Geometry: see drawing. Coordinates: mm, zero at the bounding-box minimum. A direction names the side the tool comes from. Round coordinates to 2 decimals unless told otherwise and drop trailing zeros. Loops run counter-clockwise (first coordinate to the right, second up) from the corner with the lowest first, then second, coordinate; pieces in that order, holes last.
(1) First-contact query: pin 1 Ø1.5 at (y, z) = (4, 6) entering from +X; pin 2 Ø6 at (x, z) = (7.5, 14.5) entering from -Y; pin 3 Ø1 at (x, z) = (1.5, 9.5) entering from +Y; pin 4 Ø1 at (x, z) = (7.5, 10.5) entering from -Y. Flat tips, straight axial feed; report the tip coordinate or a pass-through.
(2) Mould query, pull axis Y, two halves, no side actions, for the marked faces 3, 4, 5 and 6. Classes: pulls with the +Y half, pulls with the -Y half, needs draft (parallel to the pull), parting line crosses it, or undercut.
(3) Set-up query: the marked faces 1 and 2. Return all of +Z, -Z, +X, -X, +Y, -Y with unobstructed straight access to the full face (end or side cutting, diameter ignored); none if empty.
(4) Section C-C, the plane z = 6.25. Return the cut outline in (x, y), plus the area to 3 significant figures.
(5) Material intervals for probe 1 along Y at (x, z) = (5, 4.75); probe 2 along Y at (x, z) = (5, 9.75); probe 3 along Z at (x, y) = (3.5, 9), sorted ascending.
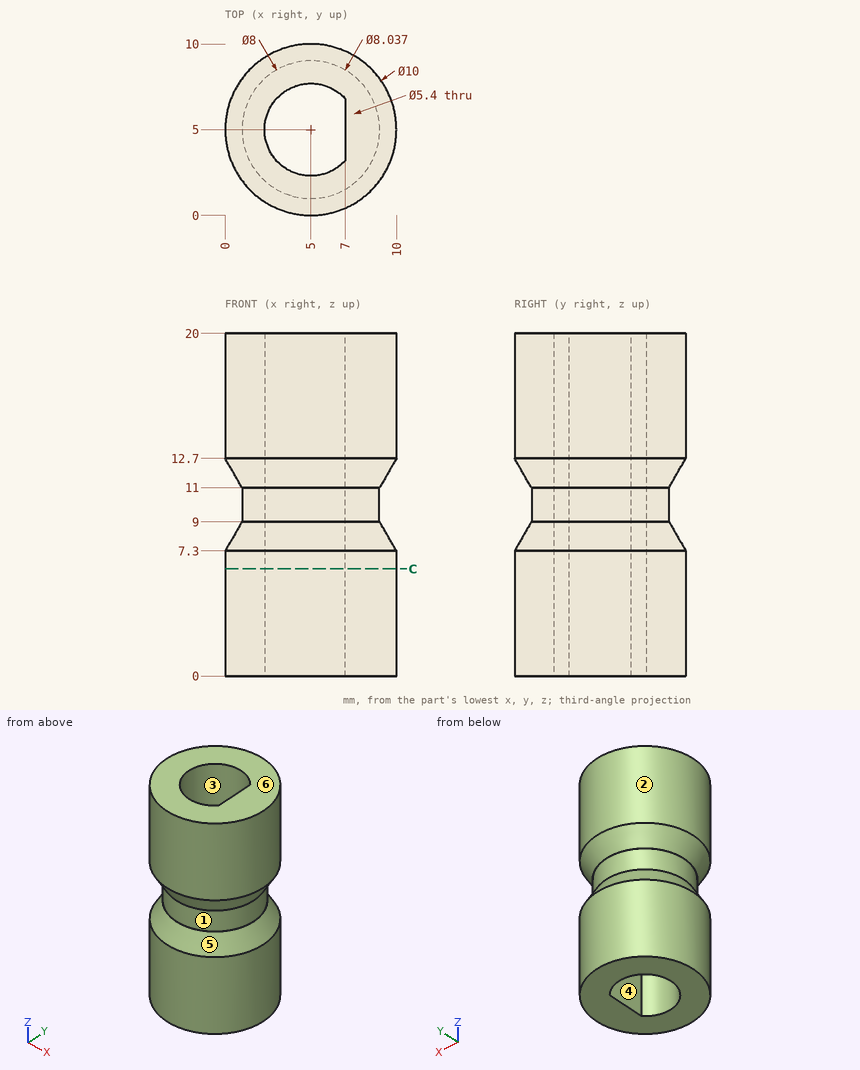
Output values:
1. pin 1: stops at x = 9.99
1. pin 2: stops at y = 0
1. pin 3: stops at y = 7.65
1. pin 4: stops at y = 1.54
2. face 3: undercut
2. face 4: undercut
2. face 5: parting line crosses it
2. face 6: needs draft
3. face 1: none
3. face 2: +Z, -Z
4. outline: circle Ø10 at (5, 5); hole (7, 3.19) - (7, 6.81) arc R2.7 ccw (long way) to start
4. area: 57.4 mm2
5. probe 1: y = 0 to 2.3, 7.7 to 10
5. probe 2: y = 1 to 2.3, 7.7 to 9
5. probe 3: z = 0 to 8.56, 11.44 to 20
